from build123d import *

# Parameters (mm, degrees)
BOSS_EXTRUDE1_DEPTH      = 1.5875
BOSS_EXTRUDE1_DEPTH_BACK = 1.5875
FILLET1_R                = 1.524
BOSS_EXTRUDE2_DEPTH      = 0.89581
BOSS_EXTRUDE2_DEPTH_BACK = 0.89581
FILLET2_R                = 1.016


with BuildPart() as part:
    # Sketch1 → Boss-Extrude1 (new, two sides: drawn at the far end of the back side and taken through both)
    with BuildSketch(Plane(origin=(0, 0, 0), x_dir=(1, 0, 0), z_dir=(0, 1, 0)).offset(-BOSS_EXTRUDE1_DEPTH_BACK)):
        with BuildLine():
            Line((-0.068296764, 6.214618695), (-0.068296764, 8.723993601))
            Line((-0.068296764, 8.723993601), (-0.895808533, 8.723993601))
            add(Edge.make_bspline(
                [(-0.895808533, 8.723993601), (-0.895808533, 4.54222596), (-1.588668774, 2.219313027), (-2.088196173, 1.337696034), (0, 0.766240154)],
                knots=[0, 0, 0, 0, 0, 1, 1, 1, 1, 1], degree=4))
            add(Edge.make_bspline(
                [(0.895808533, 8.723993601), (0.895808533, 4.54222596), (1.588668774, 2.219313027), (2.088196173, 1.337696034), (0, 0.766240154)],
                knots=[0, 0, 0, 0, 0, 1, 1, 1, 1, 1], degree=4))
            Line((0.895808533, 8.723993601), (0.068296764, 8.723993601))
            Line((0.068296764, 8.723993601), (0.068296764, 6.214618695))
            add(Edge.make_bspline(
                [(0.690807422, 2.606475487), (0.218071276, 3.482132924), (0.068296764, 6.214618695)],
                knots=[0, 0, 0, 1, 1, 1], degree=2))
            ThreePointArc((0.690807422, 2.606475487), (0, 1.52287153), (-0.690807422, 2.606475487))
            add(Edge.make_bspline(
                [(-0.690807422, 2.606475487), (-0.217222133, 3.738734236), (-0.068296764, 6.214618695)],
                knots=[0, 0, 0, 1, 1, 1], degree=2))
        make_face()
    extrude(amount=BOSS_EXTRUDE1_DEPTH + BOSS_EXTRUDE1_DEPTH_BACK)

    # Fillet1
    fillet1_edges = [part.edges().sort_by_distance(p)[0] for p in [
        (0, -0.79375, -0.766240154),
    ]]
    fillet(fillet1_edges, radius=FILLET1_R)

    # Sketch2 → Boss-Extrude2 (add, two sides: drawn at the far end of the back side and taken through both)
    with BuildSketch(Plane(origin=(0, 0, 0), x_dir=(0, 0, -1), z_dir=(1, 0, 0)).offset(-BOSS_EXTRUDE2_DEPTH_BACK)):
        Polygon((8.723993601, 1.5875), (8.723993601, -1.5875), (8.723993601, -23.8125), (9.739993601, -23.8125), (9.739993601, 1.5875), align=None)
    extrude(amount=BOSS_EXTRUDE2_DEPTH + BOSS_EXTRUDE2_DEPTH_BACK)

    # Fillet2
    fillet2_edges = [part.edges().sort_by_distance(p)[0] for p in [
        (0, 1.5875, -9.739993601),
        (0.482052648, -1.5875, -8.723993601),
        (-0.482052648, -1.5875, -8.723993601),
    ]]
    fillet(fillet2_edges, radius=FILLET2_R - 0.0001)  # a hair under: the kernel refuses the full size


solid = part.part
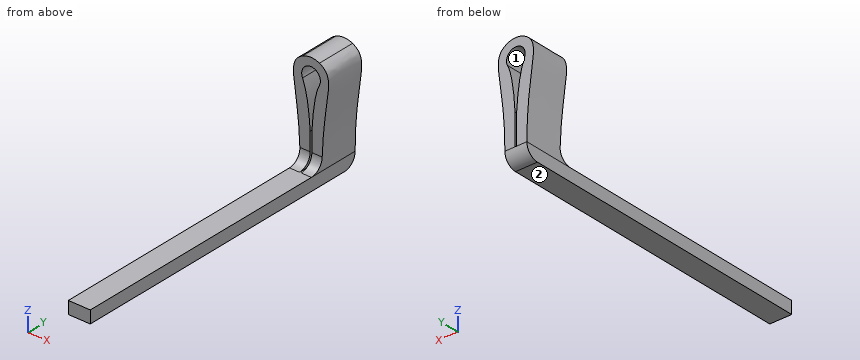
The model under review builds one solid part; all positions refer to its coordinate system, in mm. Face numbers are marked on the shaded views. Give positions to 0.01 mm unless a question says otherwise; leave off trailing zeros. Order: outer loops, then holes, each group sorted by start corner. A loop starts at its lowest first (then second) coordinate and runs counter-clockwise, first axis right, second up. Notation, with made-up numbers: M 45,-1 L 58,-1 A21 cw 58,25 Z; hole C 54,28 d5. An arc over 180 degrees is marked long. Answer in a Markdown table with one row per item. Add a question column.
1. Add section A-A on y = -4.25. State the section outline as (x, z) points, plus the area to 3 significant figures.
2. Mouldability with a two-part tool opening along X and no side actions: class the marked faces 1 and 2 as released by +X, released by -X, zero draft, split by the parting line, or undercut.
3. To check wall thickness, follow line 1 along Z through (x, y) = (0, -0.8); line 2 along Z through (x, y) = (0.6, -9); line 3 along Y through (x, z) = (0.85, -4.5). State the ranges of each line that lie inside material, in increasing order.
4. For pin 1 Ø1.5 at (x, z) = (0.5, -4.5) entering from -Y; pin 2 Ø1.5 at (x, y) = (1, -17) entering from -Z; pin 3 Ø3 at (y, z) = (0, -7) entering from -X; pin 4 Ø2 at (y, z) = (-0.5, -8) entering from +X, all flat-tipped, find the tip position at first contact; note any pin that passes through.
The answers:
| question | item | result |
|---|---|---|
| 1 | outline | M -0.9,-9.74 L 0.9,-9.74 L 0.9,-8.72 L -0.9,-8.72 Z |
| 1 | area | 1.82 mm2 |
| 2 | face 1 | undercut |
| 2 | face 2 | zero draft |
| 3 | line 1 | -9.74 to -8.72, -1.52 to -0.85 |
| 3 | line 2 | -9.74 to -8.72 |
| 3 | line 3 | -1.59 to 1.59 |
| 4 | pin 1 | y = -1.59 |
| 4 | pin 2 | z = -9.74 |
| 4 | pin 3 | x = -1.06 |
| 4 | pin 4 | x = 0.94 |
